Autodesk Inventor part; units mm, degrees
ref_plane "YZ Plane" through (0, 0, 0) normal (1, 0, 0) x (0, 1, 0)
ref_plane "XZ Plane" through (0, 0, 0) normal (0, 1, 0) x (-1, 0, 0)
ref_plane "XY Plane" through (0, 0, 0) normal (0, 0, 1) x (1, 0, 0)
ref_plane "РабПлоскость1" through (-276.9669, -64.4178, 0) normal (0, 0, 1) x (0.9934395, -0.1143588, 0)
sketch "Эскиз1" plane through (-276.9669, -64.4178, 0) normal (0, 0, 1) x (0.9934395, -0.1143588, 0)
  line L0 (291.0502, 248.6307) -> (221.0654, 248.6307) construction
  line L1 (221.0654, 248.6307) -> (209.9068, 234.7693) construction
  line L2 (209.9068, 234.7693) -> (196.6601, 234.7693) construction
  line L3 (196.6601, 234.7693) -> (196.6601, 175.7756) construction
  line L4 (196.6601, 175.7756) -> (196.6601, 136.8397) construction
  line L5 (196.6601, 136.8397) -> (196.6601, 100.2635) construction
  line L6 (196.6601, 100.2635) -> (185.4513, 58.9679) construction
  line L7 (185.4513, 58.9679) -> (192.5305, 32.4207) construction
  line L8 (192.5305, 32.4207) -> (238.9418, -16.2312) construction
  line L9 (238.9418, -16.2312) -> (291.0502, -35.7278) construction
  spline S0 degree 4 poles (291.0502, 248.6307) (221.0654, 248.6307) (209.9068, 234.7693) (196.6601, 234.7693) (196.6601, 175.7756) (196.6601, 136.8397) (196.6601, 100.2635) (185.4513, 58.9679) (192.5305, 32.4207) (238.9418, -16.2312) (291.0502, -35.7278) knots 1 1 1 1 1 2 3 4 5 6 7 8 8 8 8 8
  line L10 (291.0502, 248.6307) -> (291.0502, -35.7278)
  line L11 (295.0502, 248.6307) -> (291.0502, 248.6307)
  line L12 (291.0502, 248.6307) -> (591.0502, 248.6307) construction
  line L13 (291.0502, 248.6307) -> (-95.7817, 248.6307)
  line L14 (295.0502, -35.7278) -> (291.0502, -35.7278)
  line L15 (291.0502, -35.7278) -> (207.0762, -35.7278)
  point P0 (267.7832, 95.6688)
extrude "Выдавливание1" add sketch "Эскиз1" along normal mid plane 4
sketch "Эскиз2" plane through (10.9482, -108.3491, 1.5) normal (0.9934395, -0.1143588, 0) x (0, 0, -1)
  line L0 (3, 0) -> (0, 0)
  line L1 (0, 0) -> (0, 59.7017)
  line L2 (-0.5, -25.0103) -> (-0.5, 259.3482)
  line L3 (3.5, 259.3482) -> (3.5, -25.0103)
  line L4 (3, 59.7017) -> (3, 119.4034)
  line L5 (0, 119.4034) -> (0, 179.1051)
  line L6 (0, 179.1051) -> (3, 179.1051)
  line L7 (3, 179.1051) -> (3, 238.8068)
  line L8 (0, 238.8068) -> (0, 298.5085)
  line L9 (0, 298.5085) -> (3, 298.5085)
  line L10 (0, 59.7017) -> (3, 59.7017)
  line L11 (3, 119.4034) -> (0, 119.4034)
  line L12 (3, 238.8068) -> (0, 238.8068)
  line L13 (0, 59.7017) -> (0, 119.4034)
  line L14 (0, 179.1051) -> (0, 238.8068)
  line L15 (3, 238.8068) -> (3, 298.5085)
  line L16 (0, 298.5085) -> (3, 298.5085)
  line L17 (0, 0) -> (3, 0)
  line L18 (3, 59.7017) -> (3, 0)
  line L19 (3, 59.7017) -> (0, 59.7017)
  line L20 (0, 119.4034) -> (3, 119.4034)
  line L21 (0, 59.7017) -> (0, 119.4034)
  line L22 (3, 179.1051) -> (0, 179.1051)
  line L23 (0, 238.8068) -> (3, 238.8068)
  line L24 (3, 238.8068) -> (3, 298.5085)
  line L25 (0, 298.5085) -> (3, 298.5085)
  line L26 (0, 238.8068) -> (0, 298.5085)
  line L27 (3, 179.1051) -> (3.5, 179.1051)
  line L28 (3, 119.4034) -> (3.5, 119.4034)
  line L29 (3.5, 179.1051) -> (3.5, 119.4034)
  line L30 (0, 179.1051) -> (-0.5, 179.1051)
  line L31 (-0.5, 179.1051) -> (-0.5, 119.4034)
  line L32 (0, 119.4034) -> (-0.5, 119.4034)
  line L33 (3, 59.7017) -> (3.5, 59.7017)
  line L34 (3.5, 59.7017) -> (3.5, 0)
  line L35 (3, 0) -> (3.5, 0)
  line L36 (0, 0) -> (-0.5, 0)
  line L37 (-0.5, 0) -> (-0.5, 59.7017)
  line L38 (-0.5, 59.7017) -> (0, 59.7017)
  point P0 (1.5, 106.3863)
  point P1 (3.5, -25.0103)
  point P2 (3, 59.7017)
extrude "Выдавливание2" add sketch "Эскиз2" along normal blind 4 contours L0 L1 L10 L18 | L18 L33 L3 L35 | L36 L2 L38 L1 | L11 L5 L6 L27 L3 L28 | L32 L2 L30 L5
sketch "Эскиз3" plane through (-276.9669, -64.4178, 0) normal (0, 0, 1) x (0.9934395, -0.1143588, 0)
  point P0 (267.7832, 95.6688)
sketch "Эскиз4" plane through (-276.9669, -64.4178, 0) normal (0, 0, 1) x (0.9934395, -0.1143588, 0)
  line L0 (-21.9452, -13.2655) -> (34.011, -13.2655)
  line L1 (-21.9452, -13.2655) -> (34.011, -13.2655)
  line L2 (34.011, -13.2655) -> (34.011, -16.2655)
  line L3 (-21.9452, -13.2655) -> (34.011, -13.2655)
  line L4 (-21.9452, -16.2655) -> (-21.9452, -13.2655)
  line L5 (34.011, -16.2655) -> (-21.9452, -16.2655)
  line L6 (-21.9452, -16.2655) -> (-21.9452, -13.2655)
  line L7 (-69.5874, -16.2655) -> (-21.9452, -16.2655)
  line L8 (-21.9452, -13.2655) -> (-69.5874, -13.2655)
  line L9 (-69.5874, -13.2655) -> (-69.5874, -16.2655)
  line L10 (-21.9452, -13.2655) -> (-21.9452, -12.7655)
  line L11 (-21.9452, -12.7655) -> (-69.5874, -12.7655)
  line L12 (-69.5874, -12.7655) -> (-69.5874, -13.2655)
  line L13 (-69.5874, -16.2655) -> (-69.5874, -16.7655)
  line L14 (-69.5874, -16.7655) -> (-21.9452, -16.7655)
  line L15 (-21.9452, -16.7655) -> (-21.9452, -16.2655)
  point P0 (267.7832, 95.6688)
  point P1 (-66.0194, -13.2655)
  dimension "d16" = 0.5
  dimension "d17" = 0.5
extrude "Выдавливание3" cut sketch "Эскиз4" against normal through all both and the other way through all contours L4 L7 L9 L8 | L8 L12 L11 L10 | L15 L14 L13 L7
sketch "Эскиз5" plane through (-276.9669, -64.4178, 0) normal (0, 0, 1) x (0.9934395, -0.1143588, 0)
  line L0 (291.0502, 173.347) -> (291.0502, 169.347)
  line L1 (246.0502, 173.347) -> (291.0502, 173.347)
  line L2 (246.0502, 173.347) -> (246.0502, 169.347)
  line L3 (291.0502, 169.347) -> (246.0502, 169.347)
  line L4 (246.0502, 173.347) -> (246.0502, 169.347)
  line L5 (186.6761, 173.347) -> (246.0502, 173.347)
  line L6 (186.6761, 173.347) -> (186.6761, 169.347)
  line L7 (186.6761, 169.347) -> (246.0502, 169.347)
  line L8 (246.0502, 173.347) -> (246.0502, 169.347)
  line L9 (186.6761, 173.347) -> (186.6761, 173.847)
  line L10 (186.6761, 173.847) -> (246.0502, 173.847)
  line L11 (246.0502, 173.847) -> (246.0502, 173.347)
  line L12 (246.0502, 169.347) -> (246.0502, 168.847)
  line L13 (246.0502, 168.847) -> (186.6761, 168.847)
  line L14 (186.6761, 168.847) -> (186.6761, 169.347)
  point P0 (267.7832, 95.6688)
  dimension "d14" = 0.5
  dimension "d15" = 0.5
sketch "Эскиз6" plane through (-276.9669, -64.4178, -2) normal (0, 0, -1) x (-0.9934395, 0.1143588, 0)
  line L0 (16.8024, -31.0891) -> (36.8024, -31.0891)
  line L1 (36.8024, -31.0891) -> (36.8024, -46.0891)
  line L2 (36.8024, -46.0891) -> (16.8024, -46.0891)
  line L3 (16.8024, -46.0891) -> (16.8024, -31.0891)
  line L4 (-286.6513, 74.0401) -> (-286.6513, 59.0401)
  line L5 (-286.6513, 59.0401) -> (-266.6513, 59.0401)
  line L6 (-266.6513, 59.0401) -> (-266.6513, 74.0401)
  line L7 (-266.6513, 74.0401) -> (-286.6513, 74.0401)
  point P0 (-267.7832, 95.6688)
  dimension "d10" = 20
  dimension "d11" = 15
  dimension "d18" = 15
  dimension "d19" = 20
extrude "Выдавливание6" cut sketch "Эскиз6" against normal through all contours L7 L6 L5 L4
ref_plane "РабПлоскость2" through (1.8532, -16.6155, -86.2852) normal (-0.1143588, -0.9934395, 0) x (0, 0, 1)
sketch "Эскиз8" plane through (1.8532, -16.6155, -86.2852) normal (-0.1143588, -0.9934395, 0) x (0, 0, 1)
  line L0 (88.2852, 35.4303) -> (84.2852, 35.4303)
  line L1 (84.2852, 35.4303) -> (84.2852, 89.0995)
  line L2 (84.2852, 89.0995) -> (88.2852, 89.0995)
  line L3 (88.2852, 89.0995) -> (88.2852, 35.4303)
  point P0 (86.2852, 3.7412)
extrude "Выдавливание7" cut sketch "Эскиз8" along normal blind 1 and the other way blind 3
extrude "Выдавливание8" cut sketch "Эскиз5" against normal through all both and the other way through all contours L2 L7 L6 L5
properties part number "поперечная_поддержка"
Read the model definition and answer for the solid it produces. Units are mm, in the model's axes. A direction names the side the tool comes from. Give positions to 0.01 mm unless a question says otherwise; leave off trailing zeros. Answer in a Markdown table with one row per item. Add a question column.
Item 1: Determine the mould class of faces 4 (the face through (-14, 14, 2)), 5 (the face through (-56.04, -10.96, -0.03)), 6 (the face through (18.383, -78.736, 0.028)), 7 (the face through (-55.279, -7.017, -0.028)) for opening direction X: pulls with the +X half, pulls with the -X half, needs draft (parallel to the pull), parting line crosses it, or undercut.
Item 2: A flat-ended cylindrical pin translates along its axis: P1, Ø1.5, axis at y = 25, z = 0.5, coming from the +X side. Find the tip coordinate at first contact, or state that the pin passes through.
Item 3: Find the intervals of material crossed by L1, parallel to Y at x = -30.5, z = -1.15; L2, parallel to Y at x = -62, z = -1.8; L3, parallel to Y at x = -39.5, z = 1, in increasing order.
Item 4: A tool of negligible diameter and unlimited length cuts with its end or side. For faces 1 (the face through (-38.039, 78.544, 0.028)), 2 (the face through (36.083, 109.997, -0.028)), 3 (the face through (32.038, 39.884, 0.028)), from which of +Z, -Z, +X, -X, +Y, -Y can it reach the whole face along a straight path? Write none if from no direction.
Recorded:
| question | item | result |
|---|---|---|
| 1 | face 4 | needs draft |
| 1 | face 5 | undercut |
| 1 | face 6 | pulls with the +X half |
| 1 | face 7 | undercut |
| 2 | P1 | stops at x = 30.41 |
| 3 | L1 | y = -108.81 to 77.68, 81.7 to 151.46 |
| 3 | L2 | y = -77.05 to -10.27, -6.24 to 81.3 |
| 3 | L3 | y = -101.3 to -12.86, -8.83 to 78.71, 82.74 to 148.34 |
| 4 | face 1 | +Z, -Z |
| 4 | face 2 | +Z, -Z, +X |
| 4 | face 3 | +Z, -Z, +X, -Y |
